Source: CAD feature listing. Evaluate the final solid. Frame: model axes, mm. Face numbers are marked on the shaded views. A direction names the side the tool comes from. Coordinates: 2 decimals unless noted, no trailing zeros. Write each loop counter-clockwise with the first axis right and the second up, starting at its lowest first coordinate (ties: lowest second). Pieces come first, ordered by that corner, then holes. Notation, with made-up numbers: (2, -34) - (22, -34) arc R17 cw to (22, -10) - close; hole circle Ø4 at (27, -29.5). An arc over 180 degrees is marked (long way). One line per question, with ' | ' between items.
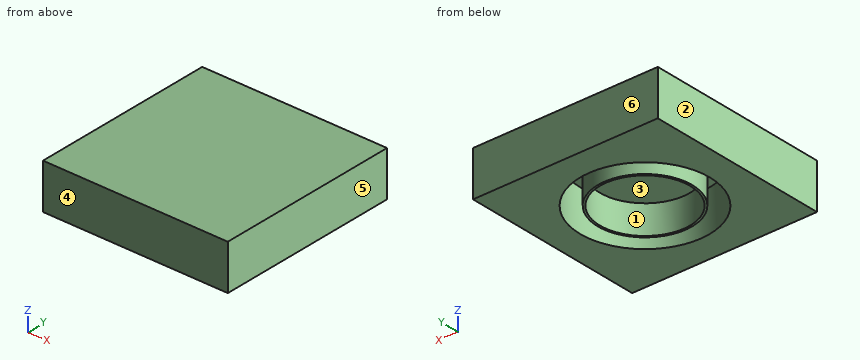
from build123d import *

# Parameters (mm, degrees)
SKIZZE1_W                       = 45
SKIZZE1_H                       = 44.9
AUFSATZ_LINEAR_AUSTRAGEN1_DEPTH = 11
SKIZZE3_R                       = 15.75
SCHNITT_LINEAR_AUSTRAGEN1_DEPTH = 10
SKIZZE7_R                       = 11.5
AUFSATZ_LINEAR_AUSTRAGEN3_DEPTH = 10
SKIZZE8_R                       = 11
SCHNITT_LINEAR_AUSTRAGEN4_DEPTH = 7


with BuildPart() as part:
    # Skizze1 → Aufsatz-Linear austragen1 (new body)
    with BuildSketch(Plane.XY):
        Rectangle(SKIZZE1_W, SKIZZE1_H)
    extrude(amount=AUFSATZ_LINEAR_AUSTRAGEN1_DEPTH)

    # Skizze3 → Schnitt-Linear austragen1 (cut)
    with BuildSketch(Plane(origin=(0, 0, 0), x_dir=(-1, 0, 0), z_dir=(0, 0, -1))):
        Circle(SKIZZE3_R)
    extrude(amount=-SCHNITT_LINEAR_AUSTRAGEN1_DEPTH, mode=Mode.SUBTRACT)

    # Skizze7 → Aufsatz-Linear austragen3 (add)
    with BuildSketch(Plane(origin=(0, 0, 0), x_dir=(-1, 0, 0), z_dir=(0, 0, -1))):
        Circle(SKIZZE7_R)
    extrude(amount=-AUFSATZ_LINEAR_AUSTRAGEN3_DEPTH)

    # Skizze8 → Schnitt-Linear austragen4 (cut)
    with BuildSketch(Plane(origin=(0, 0, 0), x_dir=(-1, 0, 0), z_dir=(0, 0, -1))):
        Circle(SKIZZE8_R)
    extrude(amount=-SCHNITT_LINEAR_AUSTRAGEN4_DEPTH, mode=Mode.SUBTRACT)


solid = part.part
Item 1: Cut plane D-D on x = -15. Return loops of the section in (y, z).
Check sheet entries:
outline: (-22.45, 0) - (-4.8, 0) - (-4.8, 10) - (4.8, 10) - (4.8, 0) - (22.45, 0) - (22.45, 11) - (-22.45, 11) - close
Item 2: Cut plane B-B on x = 0. Return loops of the section in (y, z).
Check sheet entries:
outline: (-22.45, 0) - (-15.75, 0) - (-15.75, 10) - (-11.5, 10) - (-11.5, 0) - (-11, 0) - (-11, 7) - (11, 7) - (11, 0) - (11.5, 0) - (11.5, 10) - (15.75, 10) - (15.75, 0) - (22.45, 0) - (22.45, 11) - (-22.45, 11) - close
Item 3: Pin query (flat end, axial travel): pin 1 Ø17.5 at (x, y) = (0, 0) entering from -Z. Return the tip coordinate at first contact, or that it passes through.
Check sheet entries:
pin 1: z = 7
Item 4: Cut plane A-A on z = 2. Return loops of the section in (x, y), and give its area (3 significant figures).
Check sheet entries:
outline: (-22.5, -22.45) - (22.5, -22.45) - (22.5, 22.45) - (-22.5, 22.45) - close; circle Ø23 at (0, 0); hole circle Ø31.5 at (0, 0); hole circle Ø22 at (0, 0) | area: 1,280 mm²
Item 5: Access query for the marked faces 1 and 2. Directions: +Z, -Z, +X, -X, +Y, -Y. A direction counts if a zero-diameter tool reaches every point of the face in a straight line with its end or side. Return the directions, or none.
Check sheet entries:
face 1: -Z | face 2: +Z, -Z, -X, +Y, -Y
Item 6: Mould query, pull axis Y, two halves, no side actions, for the marked faces 3, 4, 5 and 6. Classes: pulls with the +Y half, pulls with the -Y half, needs draft (parallel to the pull), parting line crosses it, or undercut.
Check sheet entries:
face 3: undercut | face 4: pulls with the -Y half | face 5: needs draft | face 6: pulls with the +Y half
Item 7: Cut plane C-C on y = 0. Return loops of the section in (x, z).
Check sheet entries:
outline: (-22.5, 0) - (-15.75, 0) - (-15.75, 10) - (-11.5, 10) - (-11.5, 0) - (-11, 0) - (-11, 7) - (11, 7) - (11, 0) - (11.5, 0) - (11.5, 10) - (15.75, 10) - (15.75, 0) - (22.5, 0) - (22.5, 11) - (-22.5, 11) - close
Item 8: Ray query, line 1 along Y through (x, z) = (0.5, 6); line 2 along Y through (x, z) = (0, 8.25); line 3 along Y through (x, z) = (-9, 8.75). Return the intervals inside material, ascending. Write a range as [from, to].
Check sheet entries:
line 1: [-22.45, -15.74], [-11.49, -10.99], [10.99, 11.49], [15.74, 22.45] | line 2: [-22.45, -15.75], [-11.5, 11.5], [15.75, 22.45] | line 3: [-22.45, -12.93], [-7.16, 7.16], [12.93, 22.45]
